Build history of the part. All positions in model axes, mm. A direction names the side the tool comes from. Round coordinates to 2 decimals unless told otherwise and drop trailing zeros. Order: outer loops, then holes, each group sorted by start corner. A loop starts at its lowest first (then second) coordinate and runs counter-clockwise, first axis right, second up. Notation, with made-up numbers: (46, 79) -> (61, 79) arc R17 cw to (61, 104) -> close; hole circle Ø3 at (-33, 1.25). An arc over 180 degrees is marked (long way). Use a Markdown table: item, result. Add a question column.
Item 1: Slice it at D-D, the plane x = -19. Give the cut face in (y, z).
Item 2: Two-plate mould, pull along Y, no slides. Class faces 6 (the face through (-0.867, 3.905, 0.493)), 7 (the face through (40, 0, 4)): released by +Y, released by -Y, zero draft, split by the parting line, or undercut.
Item 3: Slice it at A-A, the plane z = 5.5. Give the cut face in (x, y), plus the area to 3 significant figures.
Item 4: 3-axis set-ups, long thin cutter, end or side, ignore diameter. For faces 1 (the face through (-40, 0, 4)), 2 (the face through (-39, 0, 9)), 3 (the face through (-1, -28, 6)), 4 (the face through (29.67, -22.48, 0.99)), 5 (the face through (-11, 14, 1)): which of +Z, -Z, +X, -X, +Y, -Y reach the whole face in a straight line?
Item 5: Pin check, flat tips, straight feed: pin 1 (6 mm diameter, centred on x = -9.5, y = 11, fed in from -Z); pin 2 (1 mm diameter, centred on y = -1.5, z = 9, fed in from -X); pin 3 (1.6 mm diameter, centred on x = -15.5, z = 9, fed in from +Y). Stop position of each tip, or through.
Item 6: Slice it at C-C, the plane y = -21.5. Give the cut face in (x, z).
Item 7: Probe L1, parallel to Y at x = -30, z = 1.4; L2, parallel to X at y = -20, z = 1.05; L3, parallel to Y at x = -33, z = 8.5. List the from-to ranges inside material, lowest first.
Item 8: Slice it at B-B, the plane x = 30. Give the cut face in (y, z), plus the area to 3 significant figures.
from build123d import *

# Parameters (mm, degrees)
F0_W      = 80
F0_H      = 60
F1_DEPTH  = 10
F2_T      = -2
F3_W      = 80
F3_H      = 60
F3_W_2    = 77.999998
F3_H_2    = 57.999998
F4_DEPTH  = 2
F5_R      = 2.5
F6_DEPTH  = 25
F7_R      = 4
F8_DEPTH  = 1
F10_COUNT = 3


with BuildPart() as f1:
    # F0 (on Top) → F1 (new body)
    with BuildSketch(Plane.XY):
        Rectangle(F0_W, F0_H)
    extrude(amount=F1_DEPTH)

    # F2
    f2_openings = [f1.faces().sort_by_distance(p)[0] for p in [
        (0, 0, 10),
    ]]
    offset(amount=F2_T, openings=f2_openings)

    # F3 (on face) → F4 (cut)
    with BuildSketch(Plane.XY.offset(10)):
        Rectangle(F3_W, F3_H)
        Rectangle(F3_W_2, F3_H_2, mode=Mode.SUBTRACT)
    extrude(amount=-F4_DEPTH, mode=Mode.SUBTRACT)

    # F5 (on face) → F6 (cut)
    with BuildSketch(Plane(origin=(0, 0, 0), x_dir=(1, 0, 0), z_dir=(0, 0, -1))):
        with Locations((-30, 20)):
            Circle(F5_R)
        with Locations((30, -20)):
            Circle(F5_R)
        with Locations((30, 20)):
            Circle(F5_R)
        with Locations((-30, -20)):
            Circle(F5_R)
    extrude(amount=-F6_DEPTH, mode=Mode.SUBTRACT)


with BuildPart() as f8:
    # F7 (on face) → F8 (new body)
    with BuildSketch(Plane(origin=(0, 0, 0), x_dir=(1, 0, 0), z_dir=(0, 0, -1))):
        Circle(F7_R)
        with BuildLine():
            Line((-16.595718, 20.014549), (-4.069261, 5.69571))
            ThreePointArc((-4.069261, 5.69571), (-2.136589, 6.665957), (0, 7))
            Line((0, 7), (0, 26))
            ThreePointArc((0, 26), (-8.821047, 24.457905), (-16.595718, 20.014549))
        make_face()
    extrude(amount=-F8_DEPTH)


with BuildPart() as f10_1:
    # F10: instance of F8
    add(f8.part.rotate(Axis((0, 0, 0.430848), (0, 0, -1)), 1 * 360 / F10_COUNT))


with BuildPart() as f10_2:
    # F10: instance of F8
    add(f8.part.rotate(Axis((0, 0, 0.430848), (0, 0, -1)), 2 * 360 / F10_COUNT))


with BuildPart() as f1_1:
    add(f1.part)

    # F11: cut F8, F10_1, F10_2
    add(f8.part, mode=Mode.SUBTRACT)
    add(f10_1.part, mode=Mode.SUBTRACT)
    add(f10_2.part, mode=Mode.SUBTRACT)


solid = f1_1.part
Check sheet entries:
| question | item | result |
|---|---|---|
| 1 | outline | (-30, 0) -> (10.97, 0) -> (10.97, 1) -> (17.75, 1) -> (17.75, 0) -> (30, 0) -> (30, 8) -> (29, 8) -> (29, 10) -> (28, 10) -> (28, 2) -> (-28, 2) -> (-28, 10) -> (-29, 10) -> (-29, 8) -> (-30, 8) -> close |
| 2 | face 6 | undercut |
| 2 | face 7 | zero draft |
| 3 | outline | (-40, -30) -> (40, -30) -> (40, 30) -> (-40, 30) -> close; hole (-38, -28) -> (38, -28) -> (38, 28) -> (-38, 28) -> close |
| 3 | area | 544 mm2 |
| 4 | face 1 | +Z, -Z, -X, +Y, -Y |
| 4 | face 2 | +Z, -X, +Y, -Y |
| 4 | face 3 | +Z |
| 4 | face 4 | +Z, -Z |
| 4 | face 5 | -Z |
| 5 | pin 1 | z = 1 |
| 5 | pin 2 | x = -39 |
| 5 | pin 3 | y = 29 |
| 6 | outline | (-40, 0) -> (-32, 0) -> (-32, 2) -> (-38, 2) -> (-38, 10) -> (-39, 10) -> (-39, 8) -> (-40, 8) -> close; (-28, 0) -> (-14.62, 0) -> (-14.62, 1) -> (0, 1) -> (0, 0) -> (28, 0) -> (28, 2) -> (-28, 2) -> close; (32, 0) -> (40, 0) -> (40, 8) -> (39, 8) -> (39, 10) -> (38, 10) -> (38, 2) -> (32, 2) -> close |
| 7 | L1 | -30 to -22.5, -17.5 to 17.5, 22.5 to 30 |
| 7 | L2 | -40 to -32.5, -27.5 to 27.5, 32.5 to 40 |
| 7 | L3 | -29 to -28, 28 to 29 |
| 8 | outline | (-30, 0) -> (-22.5, 0) -> (-22.5, 2) -> (-28, 2) -> (-28, 10) -> (-29, 10) -> (-29, 8) -> (-30, 8) -> close; (-17.5, 0) -> (17.5, 0) -> (17.5, 2) -> (-17.5, 2) -> close; (22.5, 0) -> (30, 0) -> (30, 8) -> (29, 8) -> (29, 10) -> (28, 10) -> (28, 2) -> (22.5, 2) -> close |
| 8 | area | 128 mm2 |
